from build123d import *

# Parameters (mm, degrees)
SKETCH1_R                = 39
SKETCH1_R_2              = 26.5
BOSS_EXTRUDE1_DEPTH      = 2.25
SKETCH3_W                = 50
SKETCH3_H                = 51.5
BOSS_EXTRUDE2_DEPTH      = 2.25
BOSS_EXTRUDE4_DEPTH      = 2.25
SKETCH2_R                = 2.75
CUT_EXTRUDE1_DEPTH       = 3.25
CIRPATTERN1_COUNT        = 6
CUT_EXTRUDE2_START       = -5.5
SKETCH5_R                = 2.25
CUT_EXTRUDE2_DEPTH       = 6.5
LPATTERN1_COUNT          = 2
LPATTERN1_PITCH          = 15
LPATTERN1_COUNT_DIR2     = 2
LPATTERN1_PITCH_DIR2     = 10
LPATTERN2_COUNT          = 2
LPATTERN2_PITCH          = 15
LPATTERN2_COUNT_DIR2     = 2
LPATTERN2_PITCH_DIR2     = 10
CUT_EXTRUDE3_START       = -5.5
SKETCH7_R                = 3.25
CUT_EXTRUDE3_DEPTH       = 6.5
LPATTERN3_COUNT          = 3
LPATTERN3_PITCH          = 20
SKETCH8_R                = 3.25
CUT_EXTRUDE4_DEPTH       = 10
LPATTERN4_COUNT          = 4
LPATTERN4_PITCH          = 20
SKETCH9_W                = 27
SKETCH9_H                = 15
SKETCH9_W_2              = 4.3
SKETCH9_H_2              = 8
BOSS_EXTRUDE5_DEPTH      = 2.25
FILLET1_R                = 4
CIRPATTERN2_COUNT        = 3
CIRPATTERN2_ANGLE        = 120
FILLET1_OF_CIRPATTERN2_R = 4


with BuildPart() as part:
    # Sketch1 → Boss-Extrude1 (new body, symmetric)
    with BuildSketch(Plane(origin=(0, 0, 0), x_dir=(1, 0, 0), z_dir=(0, 1, 0))):
        Circle(SKETCH1_R)
        Circle(SKETCH1_R_2, mode=Mode.SUBTRACT)
    extrude(amount=BOSS_EXTRUDE1_DEPTH, both=True)

    # Sketch3 → Boss-Extrude2 (add, symmetric)
    with BuildSketch(Plane(origin=(0, 0, 0), x_dir=(1, 0, 0), z_dir=(0, 1, 0))):
        with Locations((0, 52.25)):
            Rectangle(SKETCH3_W, SKETCH3_H)
    extrude(amount=BOSS_EXTRUDE2_DEPTH, both=True)

    # Sketch6 → Boss-Extrude4 (add, symmetric)
    with BuildSketch(Plane(origin=(0, 0, 0), x_dir=(1, 0, 0), z_dir=(0, 1, 0))):
        Polygon((-35, 166.5), (-35, 26.5), (-39, 0), (-14.981514186, 26.5), (16.520833333, 26.5), (39, 0), (35, 26.5), (35, 166.5), align=None)
    extrude(amount=BOSS_EXTRUDE4_DEPTH, both=True)

    # Sketch2 → Cut-Extrude1 (cut, symmetric)
    with BuildSketch(Plane(origin=(0, 0, 0), x_dir=(1, 0, 0), z_dir=(0, 1, 0))):
        with Locations((0, 32.5)):
            Circle(SKETCH2_R)
    cut_extrude1 = extrude(amount=CUT_EXTRUDE1_DEPTH, both=True, mode=Mode.SUBTRACT)

    # CirPattern1: Cut-Extrude1 ×6 about axis
    cirpattern1_axis = Axis((0, 0, 0), (0, 1, 0))
    for i in range(1, CIRPATTERN1_COUNT):
        add(cut_extrude1.rotate(cirpattern1_axis, i * 360 / CIRPATTERN1_COUNT), mode=Mode.SUBTRACT)

    # Sketch5 → Cut-Extrude2 (cut)
    with BuildSketch(Plane(origin=(0, 2.25, 0), x_dir=(1, 0, 0), z_dir=(0, 1, 0)).offset(CUT_EXTRUDE2_START)):
        with Locations((0, 73)):
            Circle(SKETCH5_R)
    cut_extrude2 = extrude(amount=CUT_EXTRUDE2_DEPTH, mode=Mode.SUBTRACT)

    # LPattern1: Cut-Extrude2 2 × 2
    with Locations(*[(i * LPATTERN1_PITCH, 0, j * LPATTERN1_PITCH_DIR2) for i in range(LPATTERN1_COUNT) for j in range(LPATTERN1_COUNT_DIR2) if (i, j) != (0, 0)]):
        add(cut_extrude2, mode=Mode.SUBTRACT)

    # LPattern2: Cut-Extrude2 2 × 2
    with Locations(*[(-i * LPATTERN2_PITCH, 0, j * LPATTERN2_PITCH_DIR2) for i in range(LPATTERN2_COUNT) for j in range(LPATTERN2_COUNT_DIR2) if (i, j) != (0, 0)]):
        add(cut_extrude2, mode=Mode.SUBTRACT)

    # Sketch7 → Cut-Extrude3 (cut)
    with BuildSketch(Plane(origin=(0, 2.25, 0), x_dir=(1, 0, 0), z_dir=(0, 1, 0)).offset(CUT_EXTRUDE3_START)):
        with Locations((-15, 146.5)):
            Circle(SKETCH7_R)
        with Locations((15, 146.5)):
            Circle(SKETCH7_R)
    cut_extrude3 = extrude(amount=CUT_EXTRUDE3_DEPTH, mode=Mode.SUBTRACT)

    # LPattern3: Cut-Extrude3 ×3
    with Locations(*[(0, 0, i * LPATTERN3_PITCH) for i in range(1, LPATTERN3_COUNT)]):
        add(cut_extrude3, mode=Mode.SUBTRACT)

    # Sketch8 → Cut-Extrude4 (cut)
    with BuildSketch(Plane(origin=(0, 2.25, 0), x_dir=(1, 0, 0), z_dir=(0, 1, 0))):
        with Locations((0, 146.5)):
            Circle(SKETCH8_R)
    cut_extrude4 = extrude(amount=-CUT_EXTRUDE4_DEPTH, mode=Mode.SUBTRACT)

    # LPattern4: Cut-Extrude4 ×4
    with Locations(*[(0, 0, i * LPATTERN4_PITCH) for i in range(1, LPATTERN4_COUNT)]):
        add(cut_extrude4, mode=Mode.SUBTRACT)

    # Sketch9 → Boss-Extrude5 (add, symmetric)
    with BuildSketch(Plane(origin=(0, 0, 0), x_dir=(1, 0, 0), z_dir=(0, 1, 0))):
        with Locations((51.3, 0)):
            Rectangle(SKETCH9_W, SKETCH9_H)
        with Locations((59.65, 0)):
            Rectangle(SKETCH9_W_2, SKETCH9_H_2, mode=Mode.SUBTRACT)
    boss_extrude5 = extrude(amount=BOSS_EXTRUDE5_DEPTH, both=True)

    # Fillet1
    fillet1_edges = [part.edges().sort_by_distance(p)[0] for p in [
        (64.8, 0, 7.5),
        (64.8, 0, -7.5),
    ]]
    fillet(fillet1_edges, radius=FILLET1_R)

    # CirPattern2: Boss-Extrude5 ×3 about axis
    cirpattern2_axis = Axis((0, 0, 0), (0, -1, 0))
    for i in range(1, CIRPATTERN2_COUNT):
        add(boss_extrude5.rotate(cirpattern2_axis, i * CIRPATTERN2_ANGLE / (CIRPATTERN2_COUNT - 1)))

    # Fillet1 of CirPattern2
    fillet1_of_cirpattern2_edges = [part.edges().sort_by_distance(p)[0] for p in [
        (25.904809472, 0, 59.868446165),
        (38.895190528, 0, 52.368446165),
        (-38.895190528, 0, 52.368446165),
        (-25.904809472, 0, 59.868446165),
    ]]
    fillet(fillet1_of_cirpattern2_edges, radius=FILLET1_OF_CIRPATTERN2_R)


solid = part.part
Read the model definition and answer for the solid it produces. Units are mm, in the model's axes. A direction names the side the tool comes from. Round coordinates to 2 decimals unless told otherwise and drop trailing zeros. Write each loop counter-clockwise with the first axis right and the second up, starting at its lowest first coordinate (ties: lowest second). Pieces come first, ordered by that corner, then holes.
1. The part is cut by section C-C, the plane z = -32.5. Determine the outline of the cut face in (x, y).
2. The part is cut by section B-B, the plane x = -8.5. Determine the outline of the cut face in (y, z), then the cut area to 3 significant figures.
3. Given pin 1 Ø4 at (x, z) = (15, -63) entering from -Y; pin 2 Ø1.3 at (x, y) = (45, 0) entering from +Z; pin 3 Ø1.5 at (y, z) = (1.5, -18.5) entering from -X, each flat-ended and moving along its own axis, determine where each tip first touches the part or whether it passes through.
4. Which of the six approach directions +Z, -Z, +X, -X, +Y, -Y give full straight-line access (tool end or side, diameter ignored) to faces 1 (the face through (30.85, 0.03, 53.55)), 2 (the face through (31.184, 0.031, 39.013)), 3 (the face through (-31.184, 0.031, 39.013))?
5. Straight lines are drawn through the part: L1, parallel to X at y = 1.5, z = -107; L2, parallel to Z at x = 27.5, y = 1.5; L3, parallel to Z at x = -32, y = -1.3. For each, find the intervals that lie inside material, in ascending order.
6. The part is cut by section A-A, the plane z = -73. Determine the outline of the cut face in (x, y), then the cut area to 3 significant figures.
7. The part is cut by section D-D, the plane z = 0. Determine the outline of the cut face in (x, y), then the cut area to 3 significant figures.
Values:
1. outline: (-35, -2.25) - (-2.75, -2.25) - (-2.75, 2.25) - (-35, 2.25) - close; (2.75, -2.25) - (35, -2.25) - (35, 2.25) - (2.75, 2.25) - close
2. outline: (-2.25, -166.5) - (2.25, -166.5) - (2.25, -25.1) - (-2.25, -25.1) - close; (-2.25, 25.1) - (2.25, 25.1) - (2.25, 38.06) - (-2.25, 38.06) - close
2. area: 695 mm2
3. pin 1: passes through
3. pin 2: stops at z = 7.5
3. pin 3: stops at x = -36.32
4. face 1: +Y, -Y
4. face 2: +X, +Y, -Y
4. face 3: -X, +Y, -Y
5. L1: x = -35 to -18.21, -11.79 to -3.21, 3.21 to 11.79, 18.21 to 35
5. L2: z = -166.5 to -18.92, -13.58 to 13.58, 18.92 to 27.65, 32.63 to 50.52, 55.48 to 58.4
5. L3: z = -166.5 to 22.29, 40.43 to 47.92, 52.89 to 56.35
6. outline: (-35, -2.25) - (-17.25, -2.25) - (-17.25, 2.25) - (-35, 2.25) - close; (-12.75, -2.25) - (-2.25, -2.25) - (-2.25, 2.25) - (-12.75, 2.25) - close; (2.25, -2.25) - (12.75, -2.25) - (12.75, 2.25) - (2.25, 2.25) - close; (17.25, -2.25) - (35, -2.25) - (35, 2.25) - (17.25, 2.25) - close
6. area: 254 mm2
7. outline: (-39, -2.25) - (-26.5, -2.25) - (-26.5, 2.25) - (-39, 2.25) - close; (26.5, -2.25) - (57.5, -2.25) - (57.5, 2.25) - (26.5, 2.25) - close; (61.8, -2.25) - (64.8, -2.25) - (64.8, 2.25) - (61.8, 2.25) - close
7. area: 209 mm2
